Design review of the part built by this model. Coordinates are the model's own, in mm. A direction names the side the tool comes from. Coordinates: 2 decimals unless noted, no trailing zeros. Write each loop counter-clockwise with the first axis right and the second up, starting at its lowest first coordinate (ties: lowest second). Pieces come first, ordered by that corner, then holes. Notation, with made-up numbers: M 34,-2 L 90,-2 A21 cw 90,17 Z; hole C 2.25,-7.5 d4. An arc over 180 degrees is marked long. One line per question, with ' | ' between items.
from build123d import *

# Parameters (mm, degrees)
CYLINDER065_R            = 0.5
CYLINDER065_DEPTH        = 10
ARRAY016_COUNT           = 4
ARRAY016_PLACEMENT_ANGLE = 28
CYLINDER060_R            = 4.55
CYLINDER060_DEPTH        = 10
CYLINDER059_R            = 3.9
CYLINDER059_DEPTH        = 10
CYLINDER063_R            = 1.5
CYLINDER063_DEPTH        = 10
ARRAY018_X_COUNT         = 2
ARRAY018_X_PITCH         = 21
ARRAY018_Y_COUNT         = 2
ARRAY018_Y_PITCH         = 8
BOX008_W                 = 25
BOX008_H                 = 12
BOX008_DEPTH             = 2
FILLET008_R              = 2


with BuildPart() as array016:
    # Cylinder065 → Cylinder065 (new body)
    with BuildSketch(Plane(origin=(6, 2, 0), x_dir=(1, 0, 0), z_dir=(0, 0, 1))):
        Circle(CYLINDER065_R)
    extrude(amount=CYLINDER065_DEPTH)

    # Array016: Array016 ×4 about axis
    array016_axis = Axis((0, 0, 0), (0, 0, 1))


with BuildPart() as array016_1:
    add(array016.part)
    for i in range(1, ARRAY016_COUNT):
        add(array016.part.rotate(array016_axis, i * 360 / ARRAY016_COUNT))


with BuildPart() as array016_2:
    # Array016 placement: moved
    add(array016_1.part.rotate(Axis((0, 0, 0), (0, 0, 1)), ARRAY016_PLACEMENT_ANGLE))


with BuildPart() as mountplatelip005:
    # Cylinder060 → Cylinder060 (new body)
    with BuildSketch(Plane.XY.offset(0.6)):
        Circle(CYLINDER060_R)
    extrude(amount=CYLINDER060_DEPTH)


with BuildPart() as mountplateinnerhole004:
    # Cylinder059 → Cylinder059 (new body)
    with BuildSketch(Plane.XY):
        Circle(CYLINDER059_R)
    extrude(amount=CYLINDER059_DEPTH)


with BuildPart() as fusion020:
    # Cylinder063 → Cylinder063 (new body)
    with BuildSketch(Plane.XY):
        Circle(CYLINDER063_R)
    extrude(amount=CYLINDER063_DEPTH)

    # Array018 X: Fusion020 ×2


with BuildPart() as fusion020_1:
    add(fusion020.part)
    with Locations(*[(i * ARRAY018_X_PITCH, 0, 0) for i in range(1, ARRAY018_X_COUNT)]):
        add(fusion020.part)

    # Array018 Y: Fusion020 ×2


with BuildPart() as fusion020_2:
    add(fusion020_1.part)
    with Locations(*[(0, i * ARRAY018_Y_PITCH, 0) for i in range(1, ARRAY018_Y_COUNT)]):
        add(fusion020_1.part)


with BuildPart() as fusion020_3:
    # Array018 placement: moved
    add(fusion020_2.part.moved(Location((-10.5, -4, 0))))

    # Fusion020: union Array016, MountPlateLip005, MountPlateInnerHole004
    add(array016_2.part)
    add(mountplatelip005.part)
    add(mountplateinnerhole004.part)


with BuildPart() as backplate:
    # Box008 → Box008 (new body)
    with BuildSketch(Plane(origin=(-12.5, -6, 0), x_dir=(1, 0, 0), z_dir=(0, 0, 1))):
        with Locations((12.5, 6)):
            Rectangle(BOX008_W, BOX008_H)
    extrude(amount=BOX008_DEPTH)

    # Fillet008
    fillet008_edges = [backplate.edges().sort_by_distance(p)[0] for p in [
        (-12.5, -6, 1),
        (-12.5, 6, 1),
        (12.5, -6, 1),
        (12.5, 6, 1),
    ]]
    fillet(fillet008_edges, radius=FILLET008_R)

    # Cut023: cut Fusion020
    add(fusion020_3.part, mode=Mode.SUBTRACT)


with BuildPart() as backplate_1:
    # Cut023 placement: moved
    add(backplate.part.moved(Location((0, 2, 0))))


solid = backplate_1.part
1. Tool access review of faces 1 (the face through (-12.5, 2, 1)), 2 (the face through (-0.99, -2.44, 1.29)): name each direction out of +Z, -Z, +X, -X, +Y, -Y from which nothing blocks a thin tool from reaching the whole face with its end or side.
Answer sheet:
face 1: +Z, -Z, -X, +Y, -Y | face 2: +Z
2. Insertion check: pin 1 Ø2.5 at (x, y) = (-10.5, 6) entering from -Z. The pin has a flat end and moves straight along its axis. Give the tip position at first contact, or say it passes through.
Answer sheet:
pin 1: through
3. Draft analysis for pull direction X (two halves, no side actions). For faces 3 (the face through (-3, 6, 2)), 4 (the face through (12.5, 2, 1)), 5 (the face through (-0.845, -1.807, 0.296)), state which applies: pulls with the +X half, pulls with the -X half, needs draft (parallel to the pull), parting line crosses it, or undercut.
Answer sheet:
face 3: needs draft | face 4: pulls with the +X half | face 5: undercut
4. Take a section at B-B (x = -10.25). Write out the cut boundary in (y, z).
Answer sheet:
outline: M -4,0 L -3.48,0 L -3.48,2 L -4,2 Z; M -0.52,0 L 4.52,0 L 4.52,2 L -0.52,2 Z; M 7.48,0 L 8,0 L 8,2 L 7.48,2 Z
5. Take a section at C-C (x = -2). Write out the cut boundary in (y, z).
Answer sheet:
outline: M -4,0 L -1.35,0 L -1.35,0.6 L -2.09,0.6 L -2.09,2 L -4,2 Z; M 5.35,0 L 8,0 L 8,2 L 6.09,2 L 6.09,0.6 L 5.35,0.6 Z
6. To check wall thickness, follow line 1 along X through (y, z) = (-1, 0.55); line 2 along Y through (x, z) = (10.5, 1.1); line 3 along X through (y, z) = (7, 1.3). State the ranges of each line that lie inside material, in increasing order. Write a range as [from, to].
Answer sheet:
line 1: [-12.5, -11.62], [-9.38, -2.49], [2.49, 9.38], [11.62, 12.5] | line 2: [-4, -3.5], [-0.5, 4.5], [7.5, 8] | line 3: [-12.23, -11.62], [-9.38, 4.08], [4.63, 9.38], [11.62, 12.23]
7. Take a section at A-A (y = 2). Write out the cut boundary in (x, z).
Answer sheet:
outline: M -12.5,0 L -3.9,0 L -3.9,0.6 L -4.55,0.6 L -4.55,2 L -12.5,2 Z; M 3.9,0 L 12.5,0 L 12.5,2 L 4.55,2 L 4.55,0.6 L 3.9,0.6 Z
8. Take a section at D-D (z = 1.65). Count the separate pieces of the cut face and the enclosed holes in it, then the cut area to 3 significant figures.
Answer sheet:
separate pieces: 1 | enclosed holes: 9 | area: 200 mm^2
